Read the model definition and answer for the solid it produces. Units are mm, in the model's axes. A direction names the side the tool comes from. Coordinates: 2 decimals unless noted, no trailing zeros. Write each loop counter-clockwise with the first axis right and the second up, starting at its lowest first coordinate (ties: lowest second). Pieces come first, ordered by that corner, then holes. Notation, with made-up numbers: (-25, -11.75) -> (14, -11.75) arc R21 ccw to (14, 14.25) -> close; hole circle Ø8 at (-7, -23.5). An arc over 180 degrees is marked (long way). Return JSON: item names as keys, results as strings.
from build123d import *

# Parameters (mm, degrees)
F2_SIZE = 1.016
F3_SIZE = 1.016
F4_SIZE = 1.016
F5_SIZE = 1.016
F6_SIZE = 1.016
F7_SIZE = 1.016
F8_SIZE = 1.016


with BuildPart() as f1:
    # F0 (on Front) → F1 (revolve)
    with BuildSketch(Plane.XZ):
        Polygon((-80.1369994879, 0), (-80.1369994879, -15.3696453199), (73.2790008187, -15.3696453199), (73.2790008187, 0), (53.9750047028, 0), (53.9750047028, 9.5223551616), (29.3370001018, 9.5223551616), (29.3370001018, 21.2063547224), (-20.7010004669, 21.2063547224), (-20.7010004669, 28.0643533915), (-33.1469997764, 28.0643533915), (-33.1469997764, 15.6183550134), (-61.0870011151, 15.6183550134), (-61.0870011151, 0), align=None)
    revolve(axis=Axis((-3.302000463, 0, -18.16364564), (1, 0, 0)))

    # F2
    f2_edges = [f1.edges().sort_by_distance(p)[0] for p in [
        (-80.136999, 0, -36.327291),
    ]]
    chamfer(f2_edges, length=F2_SIZE)

    # F3
    f3_edges = [f1.edges().sort_by_distance(p)[0] for p in [
        (-61.087001, 0, -51.945646),
    ]]
    chamfer(f3_edges, length=F3_SIZE)

    # F4
    f4_edges = [f1.edges().sort_by_distance(p)[0] for p in [
        (-33.147, 0, -64.391645),
    ]]
    chamfer(f4_edges, length=F4_SIZE)

    # F5
    f5_edges = [f1.edges().sort_by_distance(p)[0] for p in [
        (-20.701, 0, -64.391645),
    ]]
    chamfer(f5_edges, length=F5_SIZE)

    # F6
    f6_edges = [f1.edges().sort_by_distance(p)[0] for p in [
        (29.337, 0, -57.533646),
    ]]
    chamfer(f6_edges, length=F6_SIZE)

    # F7
    f7_edges = [f1.edges().sort_by_distance(p)[0] for p in [
        (53.975005, 0, -45.849646),
    ]]
    chamfer(f7_edges, length=F7_SIZE)

    # F8
    f8_edges = [f1.edges().sort_by_distance(p)[0] for p in [
        (73.279001, 0, -36.327291),
    ]]
    chamfer(f8_edges, length=F8_SIZE)


solid = f1.part
1. For a pull along Z with two mould halves and no side action, classify faces 4 (the face through (-2.36, -0.84, -15.5)), 5 (the face through (73, 17, -22)), 6 (the face through (-33.147, 3, -52)) as +Z half, -Z half, draft (parallel to the pull), parting line (faces both ways), or undercut.
Taken from the geometry:
{"face 4": "undercut", "face 5": "parting line", "face 6": "draft"}
2. The part is cut by section A-A (x = -43). Determine the outline of the cut face in (y, z), then the cut area to 3 significant figures.
Taken from the geometry:
{"outline": "circle Ø67.56 at (0, -18.16); hole circle Ø5.59 at (0, -18.16)", "area": "3,560 mm2"}
3. Flat-ended cylindrical pins translate along their axes: pin 1 Ø1 at (x, z) = (-47.5, 12.5) entering from -Y; pin 2 Ø1.5 at (x, z) = (28.5, 11.5) entering from +Y; pin 3 Ø8 at (x, z) = (17.5, 13) entering from +Y. Find the tip coordinate at first contact, or state that the pin passes through.
Taken from the geometry:
{"pin 1": "stops at y = -15.21", "pin 2": "stops at y = 26.7", "pin 3": "stops at y = 28.5"}
4. A tool of negligible diameter and unlimited length cuts with its end or side. For faces 1 (the face through (-27, 45.13, -28.18)), 2 (the face through (-20.701, -40, -21)), 3 (the face through (-46.797, -1.485, -51.913)), from which of +Z, -Z, +X, -X, +Y, -Y can it reach the whole face along a straight path? Write none if from no direction.
Taken from the geometry:
{"face 1": "+X, -X", "face 2": "+X", "face 3": "-X"}
5. Consider L1, parallel to Z at x = 38, y = 0; L2, parallel to Z at x = -10, y = 0; L3, parallel to X at y = -7, z = 12. Determine where each line is inside the solid, lowest interval first.
Taken from the geometry:
{"L1": "z = -45.85 to -20.96, -15.37 to 9.52", "L2": "z = -57.53 to -20.96, -15.37 to 21.21", "L3": "x = -61.09 to 29.34"}
6. The part is cut by section B-B (x = -63). Determine the outline of the cut face in (y, z).
Taken from the geometry:
{"outline": "circle Ø36.33 at (0, -18.16); hole circle Ø5.59 at (0, -18.16)"}
